For this review, take the finished solid that the model builds, in its own axes (mm). A direction names the side the tool comes from. Round coordinates to 2 decimals unless told otherwise and drop trailing zeros. Loops run counter-clockwise (first coordinate to the right, second up) from the corner with the lowest first, then second, coordinate; pieces in that order, holes last.
1. Consider section C-C on z = -12.5. State the section outline as (x, y) points, then the cut area to 3 significant figures.
2. To check wall thickness, follow line 1 along Y through (x, z) = (0.15, -4.25); line 2 along Z through (x, y) = (0.15, 29); line 3 along Z through (x, y) = (0.65, 32). State the ranges of each line that lie inside material, in increasing order.
3. Tool access review of faces 1 (the flat face through (0, 47.55, -10)), 2 (the flat face through (0, 46.05, -10)): name each direction out of +Z, -Z, +X, -X, +Y, -Y from which nothing blocks a thin tool from reaching the whole face with its end or side.
4. Clearance check with flat-ended pins moving along their axes: pin 1 Ø0.7 at (x, y) = (0, 12) entering from -Z; pin 2 Ø6 at (y, z) = (20, -1.5) entering from -X. State where each tip first meets the part, or that it passes through.
5. Consider section A-A on x = 0.05. State the section outline as (y, z) points.
6. Consider section B-B on y = 31.5. State the section outline as (x, z) points, then the cut area to 3 significant figures.
from build123d import *


with BuildPart() as part:
    # Sweep1: sweep along a path in Sketch2
    with BuildLine(Plane.ZY) as sweep1_path:
        Line((0, 0), (0, 44.8))
        ThreePointArc((0, 44.8), (-0.585786438, 46.214213562), (-2, 46.8))
        Line((-2, 46.8), (-17.65, 46.8))
    # Sketch1 → Sweep1 (sweep)
    with BuildSketch(Plane(origin=(0, 0, 0), x_dir=(1, 0, 0), z_dir=(0, 1, 0))):
        Polygon((0.866025404, 0), (0.433012702, 0.75), (-0.433012702, 0.75), (-0.866025404, 0), (-0.433012702, -0.75), (0.433012702, -0.75), align=None)
    sweep(path=sweep1_path.line)


solid = part.part
Resolved:
1. outline: (-0.87, 46.8) - (-0.43, 46.05) - (0.43, 46.05) - (0.87, 46.8) - (0.43, 47.55) - (-0.43, 47.55) - close
1. area: 1.95 mm2
2. line 1: y = 46.05 to 47.55
2. line 2: z = -0.75 to 0.75
2. line 3: z = -0.37 to 0.37
3. face 1: +Z, -Z, +X, -X, +Y
3. face 2: -Z, +X, -X, -Y
4. pin 1: stops at z = -0.75
4. pin 2: stops at x = -0.87
5. outline: (0, -0.75) - (44.8, -0.75) arc R1.25 cw to (46.05, -2) - (46.05, -17.65) - (47.55, -17.65) - (47.55, -2) arc R2.75 ccw to (44.8, 0.75) - (0, 0.75) - close
6. outline: (-0.87, 0) - (-0.43, -0.75) - (0.43, -0.75) - (0.87, 0) - (0.43, 0.75) - (-0.43, 0.75) - close
6. area: 1.95 mm2
